Autodesk Inventor part; units mm, degrees
ref_plane "YZ Plane" through (0, 0, 0) normal (1, 0, 0) x (0, 1, 0)
ref_plane "XZ Plane" through (0, 0, 0) normal (0, 1, 0) x (-1, 0, 0)
ref_plane "XY Plane" through (0, 0, 0) normal (0, 0, 1) x (1, 0, 0)
sketch "Sketch1" plane through (0, 0, 0) normal (0, 0, 1) x (1, 0, 0)
  line L0 (-391.16, 0) -> (391.16, 0)
  line L1 (0, -55.88) -> (0, 335.28)
  line L2 (-101.6, 279.4) -> (101.6, 279.4)
  line L3 (101.6, 279.4) -> (279.4, 101.6)
  line L4 (279.4, 101.6) -> (279.4, 0)
  line L5 (279.4, 0) -> (-279.4, 0) construction
  line L6 (-279.4, 0) -> (-279.4, 101.6)
  line L7 (-279.4, 101.6) -> (-101.6, 279.4)
  line L8 (-279.4, 101.6) -> (279.4, 101.6) construction
  line L9 (276.225, 100.2849) -> (100.2849, 276.225)
  line L10 (100.2849, 276.225) -> (-100.2849, 276.225)
  line L11 (-100.2849, 276.225) -> (-276.225, 100.2849)
  line L12 (-276.225, 100.2849) -> (-276.225, 0)
  line L13 (276.225, 0) -> (276.225, 100.2849)
  line L14 (-279.4, 0) -> (-276.225, 0)
  line L15 (276.225, 0) -> (279.4, 0)
  point P0 (0, 0)
  point P1 (-279.4, 50.8)
  point P2 (0, 0)
  point P3 (0, 279.4)
  dimension "d0" = 558.8
  dimension "d1" = 101.6
  dimension "d2" = 45
  dimension "d3" = 203.2
  dimension "d4" = 3.175
  dimension "d5" = 3.175
  dimension "d6" = 3.175
  dimension "d7" = 3.175
extrude "Extrusion1" add sketch "Sketch1" along normal mid plane 254 contours L6 L7 L2 L1 L10 L11 L12 L0 | L13 L9 L10 L1 L2 L3 L4 L0
equation "\"d5\" = d4"
equation "\"d6\" = d4"
equation "\"d7\" = d4"
properties part number "middle shell"
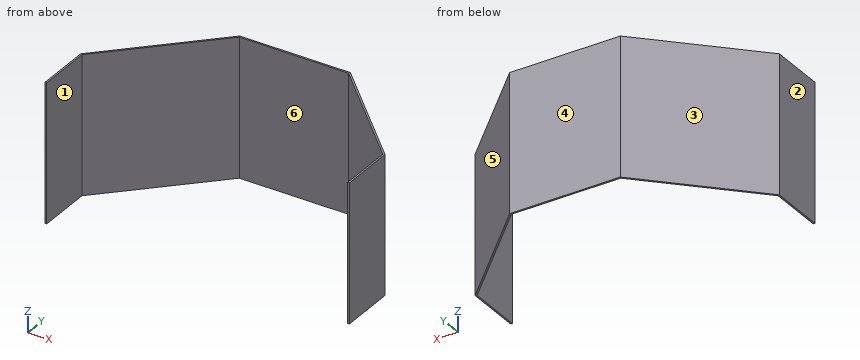
Source: CAD feature listing. Evaluate the final solid. Frame: model axes, mm. Face numbers are marked on the shaded views. A direction names the side the tool comes from. Coordinates: 2 decimals unless noted, no trailing zeros. Order: outer loops, then holes, each group sorted by start corner. A loop starts at its lowest first (then second) coordinate and runs counter-clockwise, first axis right, second up. Notation, with made-up numbers: M 62,-6.5 L 118,-6.5 A27 ccw 118,12.5 Z; hole C -1,79.25 d3. An arc over 180 degrees is marked long. Write each question's results on one line, items separated by ' | '. Start each with the question number.
1. Reachability of the marked faces 1 and 2 from +Z, -Z, +X, -X, +Y, -Y: full face, straight path, thin tool, end or side. Return the list, or none.
2. Section B-B, the plane y = 141. Return the cut outline in (x, z).
3. Section C-C, the plane x = -72.5. Return the cut outline in (y, z) (3 decimals).
4. Material intervals for L1, parallel to X at y = 57.5, z = -14 (3 decimals); L2, parallel to Y at x = 95, z = 44.5 (3 decimals); L3, parallel to X at y = 267, z = 52.5, sorted ascending.
5. Section A-A, the plane z = -51. Return the cut outline in (x, y) (3 decimals).
6. Section D-D, the plane x = -141. Return the cut outline in (y, z).
7. Draft query along X for the marked faces 3, 4, 5 and 6. Return one class per face: +X half, -X half, draft (parallel to the pull), parting line (faces both ways), or undercut.
8. Pin query (flat end, axial travel): pin 1 (12 mm diameter, centred on x = -124, z = 68, fed in from +Y); pin 2 (10 mm diameter, centred on x = -140.5, z = 31, fed in from -Y); pin 3 (10 mm diameter, centred on y = 210, z = -35.5, fed in from +X). Return the tip coordinate at first contact, or that it passes through.
Solution:
1) face 1: +Z, -Z, -Y | face 2: +Z, -Z, -X, +Y, -Y
2) outline: M -240,-127 L -235.51,-127 L -235.51,127 L -240,127 Z; M 235.51,-127 L 240,-127 L 240,127 L 235.51,127 Z
3) outline: M 276.225,-127 L 279.4,-127 L 279.4,127 L 276.225,127 Z
4) L1: -279.4 to -276.225, 276.225 to 279.4 | L2: 276.225 to 279.4 | L3: -114 to -109.51, 109.51 to 114
5) outline: M -279.4,0 L -276.225,0 L -276.225,100.285 L -100.285,276.225 L 100.285,276.225 L 276.225,100.285 L 276.225,0 L 279.4,0 L 279.4,101.6 L 101.6,279.4 L -101.6,279.4 L -279.4,101.6 Z
6) outline: M 235.51,-127 L 240,-127 L 240,127 L 235.51,127 Z
7) face 3: -X half | face 4: draft | face 5: +X half | face 6: undercut
8) pin 1: y = 263 | pin 2: y = 231.01 | pin 3: x = 176
